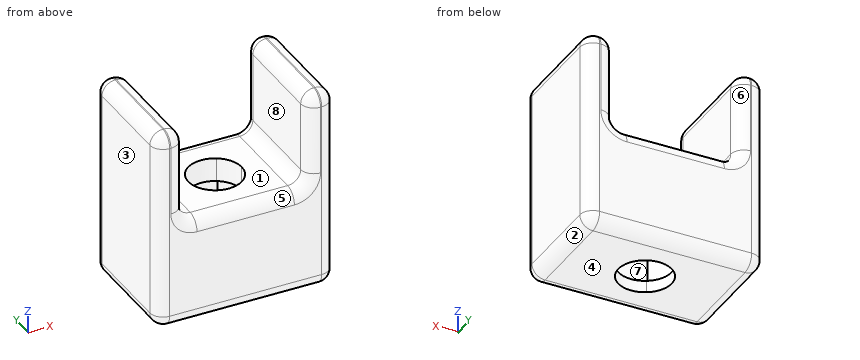
from build123d import *

# Parameters (mm, degrees)
F0_W     = 2.3
F0_H     = 8
F1_DEPTH = 10
F3_DEPTH = 17.001
F4_DEPTH = 7
F5_DEPTH = 1
F6_R     = 1.1


with BuildPart() as f1:
    # F0 (on Front) → F1 (new body)
    with BuildSketch(Plane.XZ):
        with Locations((1.15, 13)):
            Rectangle(F0_W, F0_H)
        Polygon((0, 9), (0, 0), (15, 0), (15, 9), (12.7, 9), (2.3, 9), align=None)
        with Locations((13.85, 13)):
            Rectangle(F0_W, F0_H)
    extrude(amount=F1_DEPTH)

    # F2 (on face) → F3 (cut, through all)
    with BuildSketch(Plane(origin=(0, 0, 0), x_dir=(1, 0, 0), z_dir=(0, 0, -1))):
        with BuildLine():
            Line((8.625, 3.0514428415), (6.375, 6.9485571585))
            ThreePointArc((6.375, 6.9485571585), (5.5514428415, 3.875), (8.625, 3.0514428415))
        make_face()
        with BuildLine():
            ThreePointArc((8.625, 3.0514428415), (9.4485571585, 3.875), (9.75, 5))
            ThreePointArc((9.75, 5), (8.625, 6.9485571585), (6.375, 6.9485571585))
            Line((6.375, 6.9485571585), (8.625, 3.0514428415))
        make_face()
    extrude(amount=-F3_DEPTH, mode=Mode.SUBTRACT)

    # F2 (on face) → F4 (cut)
    with BuildSketch(Plane(origin=(0, 0, 0), x_dir=(1, 0, 0), z_dir=(0, 0, -1))):
        with BuildLine():
            ThreePointArc((8.625, 3.0514428415), (5.5514428415, 3.875), (6.375, 6.9485571585))
            Line((6.375, 6.9485571585), (5.3349364905, 8.75))
            Line((5.3349364905, 8.75), (3.1698729811, 5))
            Line((3.1698729811, 5), (5.3349364905, 1.25))
            Line((5.3349364905, 1.25), (9.6650635095, 1.25))
            Line((9.6650635095, 1.25), (8.625, 3.0514428415))
        make_face()
        with BuildLine():
            ThreePointArc((6.375, 6.9485571585), (8.625, 6.9485571585), (9.75, 5))
            ThreePointArc((9.75, 5), (9.4485571585, 3.875), (8.625, 3.0514428415))
            Line((8.625, 3.0514428415), (9.6650635095, 1.25))
            Line((9.6650635095, 1.25), (11.8301270189, 5))
            Line((11.8301270189, 5), (9.6650635095, 8.75))
            Line((9.6650635095, 8.75), (5.3349364905, 8.75))
            Line((5.3349364905, 8.75), (6.375, 6.9485571585))
        make_face()
    extrude(amount=-F4_DEPTH, mode=Mode.SUBTRACT)

    # F2 (on face) → F5 (join)
    with BuildSketch(Plane(origin=(0, 0, 0), x_dir=(1, 0, 0), z_dir=(0, 0, -1))):
        with BuildLine():
            ThreePointArc((8.625, 3.0514428415), (5.5514428415, 3.875), (6.375, 6.9485571585))
            Line((6.375, 6.9485571585), (5.3349364905, 8.75))
            Line((5.3349364905, 8.75), (3.1698729811, 5))
            Line((3.1698729811, 5), (5.3349364905, 1.25))
            Line((5.3349364905, 1.25), (9.6650635095, 1.25))
            Line((9.6650635095, 1.25), (8.625, 3.0514428415))
        make_face()
        with BuildLine():
            ThreePointArc((6.375, 6.9485571585), (8.625, 6.9485571585), (9.75, 5))
            ThreePointArc((9.75, 5), (9.4485571585, 3.875), (8.625, 3.0514428415))
            Line((8.625, 3.0514428415), (9.6650635095, 1.25))
            Line((9.6650635095, 1.25), (11.8301270189, 5))
            Line((11.8301270189, 5), (9.6650635095, 8.75))
            Line((9.6650635095, 8.75), (5.3349364905, 8.75))
            Line((5.3349364905, 8.75), (6.375, 6.9485571585))
        make_face()
    extrude(amount=-F5_DEPTH)

    # F6
    f6_edges = [f1.edges().sort_by_distance(p)[0] for p in [
        (0, 0, 8.5),
        (7.5, 0, 0),
        (15, 0, 8.5),
        (13.85, 0, 17),
        (12.7, 0, 13),
        (7.5, 0, 9),
        (2.3, 0, 13),
        (1.15, 0, 17),
        (0, -10, 8.5),
        (7.5, -10, 0),
        (15, -10, 8.5),
        (13.85, -10, 17),
        (12.7, -10, 13),
        (7.5, -10, 9),
        (2.3, -10, 13),
        (1.15, -10, 17),
        (15, -5, 0),
        (15, -5, 17),
        (0, -5, 17),
        (0, -5, 0),
        (12.7, -5, 17),
        (12.7, -5, 9),
        (2.3, -5, 9),
        (2.3, -5, 17),
    ]]
    fillet(f6_edges, radius=F6_R)


solid = f1.part
Geometry: final body of the model. Coordinates: model frame, mm. Face numbers are marked on the shaded views. A direction names the side the tool comes from. Give positions to 0.01 mm unless a question says otherwise; leave off trailing zeros. Write each loop counter-clockwise with the first axis right and the second up, starting at its lowest first coordinate (ties: lowest second). Pieces come first, ordered by that corner, then holes.
(1) Access query for the marked faces 5, 6, 7 and 8. Directions: +Z, -Z, +X, -X, +Y, -Y. A direction counts if a zero-diameter tool reaches every point of the face in a straight line with its end or side. Return the directions, or none.
(2) Cut plane A-A, the plane z = 11. Return loops of the section in (x, y), then the cut area to 3 significant figures.
(3) Mould query, pull axis X, two halves, no side actions, for the marked faces 1, 2, 3 and 4. Classes: released by +X, released by -X, zero draft, split by the parting line, or undercut.
(4) First-contact query: P1, Ø4, axis at x = 1.5, y = -6.5, coming from the -Z side; P2, Ø2, axis at x = 6, y = -4, coming from the +Z side; P3, Ø8, axis at x = 9.5, z = 13, coming from the +Y side. Flat tips, straight axial feed; report the tip coordinate or a pass-through.
(5) Cut plane B-B, the plane x = 7.5. Return loops of the section in (y, z), then the cut area to 3 significant figures.
(6) Cut plane C-C, the plane z = 1.5. Return loops of the section in (x, y), then the cut area to 3 significant figures.
(7) Cut plane D-D, the plane y = -8. Return loops of the section in (x, z), then the cut area to 3 significant figures.
(8) Ray query, line 1 (X direction, y = -3.5, z = 11.25); line 2 (Z direction, x = 10.25, y = -5.5); line 3 (Z direction, x = 11, y = -7). Return the intervals inside material, ascending.
Values follow:
1. face 5: +Z, -Y
1. face 6: +Z, +Y
1. face 7: none
1. face 8: +Z, +Y, -Y
2. outline: (0, -8.9) arc R1.1 ccw to (1.1, -10) - (1.2, -10) arc R1.1 ccw to (2.3, -8.9) - (2.3, -1.1) arc R1.1 ccw to (1.2, 0) - (1.1, 0) arc R1.1 ccw to (0, -1.1) - close; (12.7, -8.9) arc R1.1 ccw to (13.8, -10) - (13.9, -10) arc R1.1 ccw to (15, -8.9) - (15, -1.1) arc R1.1 ccw to (13.9, 0) - (13.8, 0) arc R1.1 ccw to (12.7, -1.1) - close
2. area: 43.9 mm2
3. face 1: undercut
3. face 2: released by +X
3. face 3: released by -X
3. face 4: zero draft
4. P1: stops at z = 0
4. P2: stops at z = 9
4. P3: stops at y = -0.04
5. outline: (-10, 1.1) arc R1.1 ccw to (-8.9, 0) - (-7.25, 0) - (-7.25, 1) - (-8.75, 1) - (-8.75, 7) - (-7.25, 7) - (-7.25, 9) - (-8.9, 9) arc R1.1 ccw to (-10, 7.9) - close; (-2.75, 0) - (-1.1, 0) arc R1.1 ccw to (0, 1.1) - (0, 7.9) arc R1.1 ccw to (-1.1, 9) - (-2.75, 9) - (-2.75, 7) - (-1.25, 7) - (-1.25, 1) - (-2.75, 1) - close
5. area: 30.5 mm2
6. outline: (0, -8.9) arc R1.1 ccw to (1.1, -10) - (13.9, -10) arc R1.1 ccw to (15, -8.9) - (15, -1.1) arc R1.1 ccw to (13.9, 0) - (1.1, 0) arc R1.1 ccw to (0, -1.1) - close; hole (3.17, -5) - (5.33, -8.75) - (9.67, -8.75) - (11.83, -5) - (9.67, -1.25) - (5.33, -1.25) - close
6. area: 100 mm2
7. outline: (0, 1.1) arc R1.1 ccw to (1.1, 0) - (13.9, 0) arc R1.1 ccw to (15, 1.1) - (15, 15.9) arc R1.1 ccw to (13.9, 17) - (13.8, 17) arc R1.1 ccw to (12.7, 15.9) - (12.7, 10.1) arc R1.1 cw to (11.6, 9) - (3.4, 9) arc R1.1 cw to (2.3, 10.1) - (2.3, 15.9) arc R1.1 ccw to (1.2, 17) - (1.1, 17) arc R1.1 ccw to (0, 15.9) - close; hole (4.9, 1) - (10.1, 1) - (10.1, 7) - (4.9, 7) - close
7. area: 140 mm2
8. line 1: x = 0 to 2.3, 12.7 to 15
8. line 2: z = 0 to 1, 7 to 9
8. line 3: z = 0 to 9
